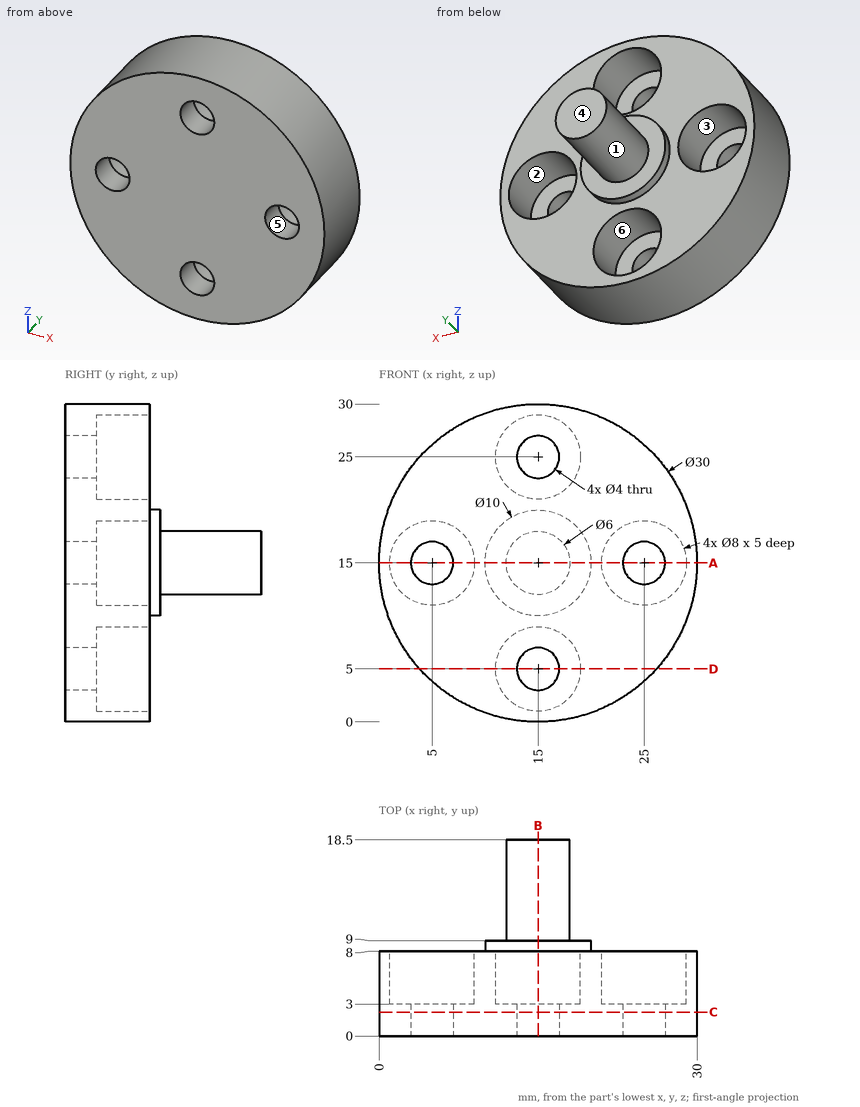
Verification items for this drawing (mm, ordinates from the low corner). A direction names the side the tool comes from. Give positions to 0.01 mm unless a question says otherwise; leave off trailing zeros. Loops run counter-clockwise (first coordinate to the right, second up) from the corner with the lowest first, then second, coordinate; pieces in that order, holes last. Notation, with made-up numbers: M -33,87.25 L -21,87.25 A28 cw -21,117.25 Z; hole C 78,22.25 d8. An arc over 180 degrees is marked long. Answer in a Markdown table with one row per item.
1) Cross-section at B-B (x = 15). Enter the section's corners in (y, z), plus the area to 3 significant figures.
Solutions:
| item | result |
|---|---|
| outline | M 0,0 L 8,0 L 8,1 L 3,1 L 3,3 L 0,3 Z; M 0,7 L 3,7 L 3,9 L 8,9 L 8,10 L 9,10 L 9,12 L 18.5,12 L 18.5,18 L 9,18 L 9,20 L 8,20 L 8,21 L 3,21 L 3,23 L 0,23 Z; M 0,27 L 3,27 L 3,29 L 8,29 L 8,30 L 0,30 Z |
| area | 203 mm^2 |
2) Depth check by flat-ended pin: pin 1 (2 mm diameter, centred on x = 5, z = 4.5, fed in from -Y); pin 2 (2.5 mm diameter, centred on x = 3.5, z = 14.5, fed in from +Y); pin 3 (9 mm diameter, centred on x = 23.5, z = 15, fed in from +Y); pin 4 (1 mm diameter, centred on x = 16.5, y = 11, fed in from +Z). Enter the tip coordinate at first touch or a pass-through.
Solutions:
| item | result |
|---|---|
| pin 1 | stops at y = 0 |
| pin 2 | stops at y = 3 |
| pin 3 | stops at y = 9 |
| pin 4 | stops at z = 17.83 |
3) Cross-section at C-C (y = 2.25). Enter the section's corners in (x, z), plus the area to 3 significant figures.
Solutions:
| item | result |
|---|---|
| outline | C 15,15 d30; hole C 5,15 d4; hole C 15,5 d4; hole C 15,25 d4; hole C 25,15 d4 |
| area | 657 mm^2 |
4) Thickness scan on line 1 (Z direction, x = 15, y = 1.5); line 2 (Z direction, x = 14.5, y = 6.75). Record the ranges inside material, lowest first.
Solutions:
| item | result |
|---|---|
| line 1 | z = 0 to 3, 7 to 23, 27 to 30 |
| line 2 | z = 0.01 to 1.03, 8.97 to 21.03, 28.97 to 29.99 |
5) Cross-section at D-D (z = 5). Enter the section's corners in (x, y).
Solutions:
| item | result |
|---|---|
| outline | M 3.82,0 L 13,0 L 13,3 L 11,3 L 11,8 L 3.82,8 Z; M 17,0 L 26.18,0 L 26.18,8 L 19,8 L 19,3 L 17,3 Z |
6) Cross-section at A-A (z = 15). Enter the section's corners in (x, y), plus the area to 3 significant figures.
Solutions:
| item | result |
|---|---|
| outline | M 0,0 L 3,0 L 3,3 L 1,3 L 1,8 L 0,8 Z; M 7,0 L 23,0 L 23,3 L 21,3 L 21,8 L 20,8 L 20,9 L 18,9 L 18,18.5 L 12,18.5 L 12,9 L 10,9 L 10,8 L 9,8 L 9,3 L 7,3 Z; M 27,0 L 30,0 L 30,8 L 29,8 L 29,3 L 27,3 Z |
| area | 203 mm^2 |
7) Tool access check on the marked faces 5 and 6. Record the directions out of +Z, -Z, +X, -X, +Y, -Y that give a thin tool (end or side, any length) a straight path to the whole face; none if there is none.
Solutions:
| item | result |
|---|---|
| face 5 | +Y, -Y |
| face 6 | +Y |
8) Mould release check, pull along X, two halves, no side actions. Record for the marked faces 1, 2, 3 and 4: released by +X, released by -X, zero draft, split by the parting line, or undercut.
Solutions:
| item | result |
|---|---|
| face 1 | split by the parting line |
| face 2 | undercut |
| face 3 | undercut |
| face 4 | zero draft |
